Design review of the part built by this model. Coordinates are the model's own, in mm. Give positions to 0.01 mm unless a question says otherwise; leave off trailing zeros. Loops run counter-clockwise (first coordinate to the right, second up) from the corner with the lowest first, then second, coordinate; pieces in that order, holes last. Notation, with made-up numbers: (-8, 18) -> (18, 18) arc R4 ccw to (18, 25) -> close; hole circle Ø1 at (75, -39). An arc over 180 degrees is marked (long way). Use a Markdown table: item, result. Add a question column.
1. To check wall thickness, follow line 1 (Y direction, x = 27.5, z = 0.95); line 2 (X direction, y = 29, z = 3.8); line 3 (Y direction, x = 33, z = 2). State the ranges of each line that lie inside material, in increasing order.
2. Add section D-D (z = 2.7). Count the separate pieces of the cut face and the enclosed holes in it, and give its area (3 significant figures).
3. Add section A-A (y = 0). State the section outline as (x, z) points.
4. For pin 1 Ø4 at (x, y) = (0, 55) entering from +Z, flat-tipped, find the tip position at first contact; note if it passes through.
5. Add section C-C (x = 21.5). State the section outline as (y, z) points.
6. Add section B-B (x = 0). State the section outline as (y, z) points, and give its area (3 significant figures).
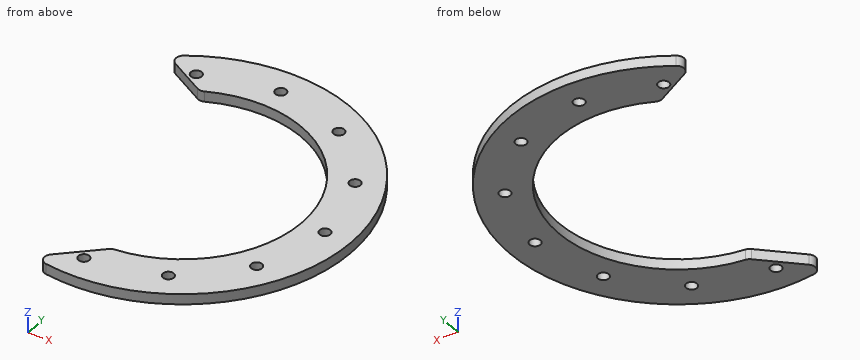
```python
from build123d import *

# Parameters (mm, degrees)
SKETCH_1_R          = 65
SKETCH_1_R_2        = 46
EXTRUDE_1_DEPTH     = 4
SKETCH_2_R          = 2.1
CUT_EXTRUDE_1_DEPTH = 4
CUT_EXTRUDE_START   = -4
CUT_EXTRUDE_2_DEPTH = 4
FILLET_1_R          = 3
CUT_EXTRUDE_START_2 = -15
CUT_EXTRUDE_3_DEPTH = 15
FILLET_2_R          = 3


with BuildPart() as part:
    # 草图1 → 凸台-拉伸1 (new body)
    with BuildSketch(Plane.XY):
        Circle(SKETCH_1_R)
        Circle(SKETCH_1_R_2, mode=Mode.SUBTRACT)
    extrude(amount=EXTRUDE_1_DEPTH)

    # 草图2 → 切除-拉伸1 (cut)
    with BuildSketch(Plane.XY.offset(4)):
        with Locations((0, 55)):
            Circle(SKETCH_2_R)
        with Locations((27.5, 47.631397208)):
            Circle(SKETCH_2_R)
        with Locations((47.631397208, 27.5)):
            Circle(SKETCH_2_R)
        with Locations((55, 0)):
            Circle(SKETCH_2_R)
        with Locations((47.631397208, -27.5)):
            Circle(SKETCH_2_R)
        with Locations((27.5, -47.631397208)):
            Circle(SKETCH_2_R)
        with Locations((0, -55)):
            Circle(SKETCH_2_R)
        with Locations((-27.5, -47.631397208)):
            Circle(SKETCH_2_R)
        with Locations((-47.631397208, -27.5)):
            Circle(SKETCH_2_R)
        with Locations((-55, 0)):
            Circle(SKETCH_2_R)
        with Locations((-47.631397208, 27.5)):
            Circle(SKETCH_2_R)
        with Locations((-27.5, 47.631397208)):
            Circle(SKETCH_2_R)
    extrude(amount=-CUT_EXTRUDE_1_DEPTH, mode=Mode.SUBTRACT)

    # 草图3 → 切除-拉伸2 (cut)
    with BuildSketch(Plane.XY.offset(4).offset(CUT_EXTRUDE_START)):
        with BuildLine():
            Line((-40.462378993, 50.870383193), (27, 15))
            Line((27, 15), (-21.728491376, -61.260694271))
            ThreePointArc((-21.728491376, -61.260694271), (-64.11139308, -10.711175351), (-40.462378993, 50.870383193))
        make_face()
    extrude(amount=CUT_EXTRUDE_2_DEPTH, mode=Mode.SUBTRACT)

    # 圆角1
    fillet_1_edges = [part.edges().sort_by_distance(p)[0] for p in [
        (-11.107555195, -44.638797224, 2),
        (-21.385147835, 40.726839456, 2),
        (-21.728491376, -61.260694271, 2),
        (-40.462378993, 50.870383193, 2),
    ]]
    fillet(fillet_1_edges, radius=FILLET_1_R)

    # 草图4 → 切除-拉伸3 (cut)
    with BuildSketch(Plane.XY.offset(4).offset(CUT_EXTRUDE_START_2)):
        with BuildLine():
            Line((-37.660954125, -86.195196375), (4.448149198, -45.784429326))
            ThreePointArc((4.448149198, -45.784429326), (-2.360891137, -45.939375192), (-9.118175919, -45.087236197))
            ThreePointArc((-9.118175919, -45.087236197), (-10.884781804, -45.266086971), (-12.24083237, -46.412390079))
            Line((-12.24083237, -46.412390079), (-37.660954125, -86.195196375))
        make_face()
    extrude(amount=CUT_EXTRUDE_3_DEPTH, mode=Mode.SUBTRACT)

    # 圆角2
    fillet_2_edges = [part.edges().sort_by_distance(p)[0] for p in [
        (-13.988029274, -63.477043386, 2),
        (4.448149198, -45.784429326, 2),
    ]]
    fillet(fillet_2_edges, radius=FILLET_2_R)


solid = part.part
```
Taken from the geometry:
| question | item | result |
|---|---|---|
| 1 | line 1 | y = -58.9 to -49.73, -45.53 to -36.87, 36.87 to 45.53, 49.73 to 58.9 |
| 1 | line 2 | x = 35.71 to 46.16, 49.1 to 58.17 |
| 1 | line 3 | y = -56 to -32.05, 32.05 to 56 |
| 2 | separate pieces | 1 |
| 2 | enclosed holes | 8 |
| 2 | area | 3,920 mm^2 |
| 3 | outline | (46, 0) -> (52.9, 0) -> (52.9, 4) -> (46, 4) -> close; (57.1, 0) -> (65, 0) -> (65, 4) -> (57.1, 4) -> close |
| 4 | pin 1 | passes through |
| 5 | outline | (-61.34, 0) -> (-40.67, 0) -> (-40.67, 4) -> (-61.34, 4) -> close; (40.67, 0) -> (61.34, 0) -> (61.34, 4) -> (40.67, 4) -> close |
| 6 | outline | (-65, 0) -> (-57.1, 0) -> (-57.1, 4) -> (-65, 4) -> close; (-52.9, 0) -> (-50.05, 0) -> (-50.05, 4) -> (-52.9, 4) -> close; (46, 0) -> (52.9, 0) -> (52.9, 4) -> (46, 4) -> close; (57.1, 0) -> (65, 0) -> (65, 4) -> (57.1, 4) -> close |
| 6 | area | 102 mm^2 |
